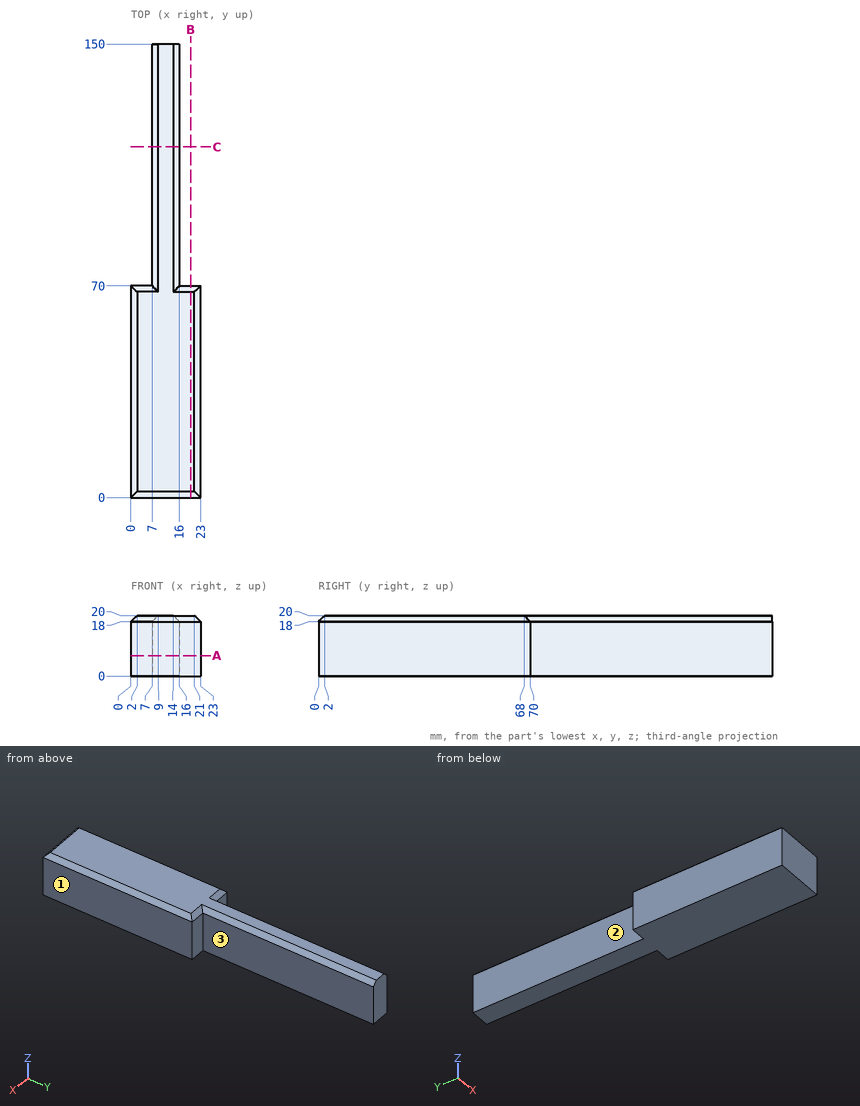
Part print with two shaded views. Sizes in mm from the minimum x, y, z corner. A direction names the side the tool comes from. Round coordinates to 2 decimals unless told otherwise and drop trailing zeros. Write each loop counter-clockwise with the first axis right and the second up, starting at its lowest first coordinate (ties: lowest second). Pieces come first, ordered by that corner, then holes. Notation, with made-up numbers: M 24.25,27.25 L 70.25,27.25 A17 ccw 70.25,38.25 Z; hole C 39.5,-18.75 d7. An arc over 180 degrees is marked long. Answer as CSV lines item,"result". Start each with the question number.
1) Band-saw the part on B-B (x = 19.75). List the corners of the cut face in (y, z).
2) Drill centre lines: L1, parallel to X at y = 135, z = 15; L2, parallel to Y at x = 4.5, z = 6.25; L3, parallel to Z at x = 18.75, y = 69. Where is each one in solid material? Low to high.
3) Band-saw the part on A-A (z = 6.75). List the corners of the cut face in (x, y), then the cut area to 3 significant figures.
4) Band-saw the part on C-C (y = 116). List the corners of the cut face in (x, z).
5) Drop flat-ended pins along their axis: pin 1 (3.5 mm diameter, centred on x = 18.5, z = 9.5, fed in from +Y); pin 2 (2 mm diameter, centred on y = 79.5, z = 11, fed in from +X); pin 3 (12 mm diameter, centred on y = 104, z = 17, fed in from -X). Give the stop position or say it passes through.
6) Which spindle directions (+Z, -Z, +X, -X, +Y, -Y) get a long thin tool onto all of the face, cutting with end or side? Do the marked faces 1, 2 and 3. Say none if no direction does.
Worked out:
1,outline,"M 0,0 L 70,0 L 70,18 L 68,20 L 2,20 L 0,18 Z"
2,L1,"7 to 16"
2,L2,"0 to 70"
2,L3,"0 to 19"
3,outline,"M 0,0 L 23,0 L 23,70 L 16,70 L 16,150 L 7,150 L 7,70 L 0,70 Z"
3,area,"2,330 mm²"
4,outline,"M 7,0 L 16,0 L 16,18 L 14,20 L 9,20 L 7,18 Z"
5,pin 1,"y = 70"
5,pin 2,"x = 16"
5,pin 3,"x = 7"
6,face 1,"+Z, -Z, +X, +Y, -Y"
6,face 2,"+Z, -Z, -X, +Y"
6,face 3,"+Z, -Z, +X, +Y"
